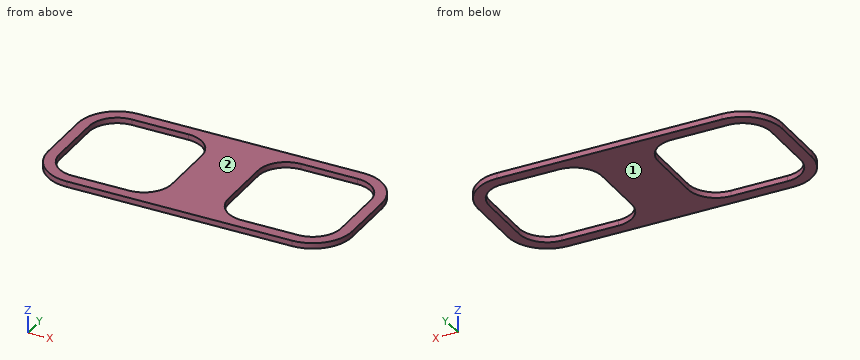
```python
from build123d import *

# Parameters (mm, degrees)
F1_DEPTH = 0.5


with BuildPart() as f1:
    # F0 (on Top) → F1 (new body)
    with BuildSketch(Plane.XY):
        with BuildLine():
            Line((-13.5, 2.5), (-13.5, 0))
            Line((-13.5, 0), (-13.5, -2.5))
            ThreePointArc((-13.5, -2.5), (-12.474874, -4.974874), (-10, -6))
            Line((-10, -6), (10, -6))
            ThreePointArc((10, -6), (12.474874, -4.974874), (13.5, -2.5))
            Line((13.5, -2.5), (13.5, 2.5))
            ThreePointArc((13.5, 2.5), (12.474874, 4.974874), (10, 6))
            Line((10, 6), (-10, 6))
            ThreePointArc((-10, 6), (-12.474874, 4.974874), (-13.5, 2.5))
        make_face()
        with BuildLine():
            Line((-2.5, 2.5), (-2.5, 0))
            Line((-2.5, 0), (-2.5, -2.5))
            ThreePointArc((-2.5, -2.5), (-3.232233, -4.267767), (-5, -5))
            Line((-5, -5), (-10, -5))
            ThreePointArc((-10, -5), (-11.767767, -4.267767), (-12.5, -2.5))
            Line((-12.5, -2.5), (-12.5, 0))
            Line((-12.5, 0), (-12.5, 2.5))
            ThreePointArc((-12.5, 2.5), (-11.767767, 4.267767), (-10, 5))
            Line((-10, 5), (-5, 5))
            ThreePointArc((-5, 5), (-3.232233, 4.267767), (-2.5, 2.5))
        make_face(mode=Mode.SUBTRACT)
        with BuildLine():
            Line((2.5, -2.5), (2.5, 0))
            Line((2.5, 0), (2.5, 2.5))
            ThreePointArc((2.5, 2.5), (3.232233, 4.267767), (5, 5))
            Line((5, 5), (10, 5))
            ThreePointArc((10, 5), (11.767767, 4.267767), (12.5, 2.5))
            Line((12.5, 2.5), (12.5, -2.5))
            ThreePointArc((12.5, -2.5), (11.767767, -4.267767), (10, -5))
            Line((10, -5), (5, -5))
            ThreePointArc((5, -5), (3.232233, -4.267767), (2.5, -2.5))
        make_face(mode=Mode.SUBTRACT)
    extrude(amount=F1_DEPTH)


solid = f1.part
```
Read the model definition and answer for the solid it produces. Units are mm, in the model's axes. Face numbers are marked on the shaded views. Round coordinates to 2 decimals unless told otherwise and drop trailing zeros. Write each loop counter-clockwise with the first axis right and the second up, starting at its lowest first coordinate (ties: lowest second). Pieces come first, ordered by that corner, then holes. Notation, with made-up numbers: (0.25, -5.5) -> (42.25, -5.5) arc R25 ccw to (42.25, 24.5) -> close; hole circle Ø10 at (79.5, 37). An arc over 180 degrees is marked (long way). Answer in a Markdown table with one row per item. Add a question column.
1) Find section B-B, the plane y = 0.5. Determine the outline of the cut face in (x, z).
2) Determine the mould class of the marked faces 1 and 2 for opening direction Z: pulls with the +Z half, pulls with the -Z half, needs draft (parallel to the pull), parting line crosses it, or undercut.
3) Find section C-C, the plane z = 0.4. Determine the outline of the cut face in (x, y).
4) Find section D-D, the plane y = 3.5. Determine the outline of the cut face in (x, z).
5) Consider line 1 (X direction, y = -1.25, z = 0.3); line 2 (Y direction, x = 7.75, z = 0.1); line 3 (X direction, y = -3.5, z = 0.1). Determine where each line is inside the solid, lowest interval first.
6) Find section A-A, the plane x = -7.5. Determine the outline of the cut face in (y, z), and give its area (3 significant figures).
Findings below:
| question | item | result |
|---|---|---|
| 1 | outline | (-13.5, 0) -> (-12.5, 0) -> (-12.5, 0.5) -> (-13.5, 0.5) -> close; (-2.5, 0) -> (2.5, 0) -> (2.5, 0.5) -> (-2.5, 0.5) -> close; (12.5, 0) -> (13.5, 0) -> (13.5, 0.5) -> (12.5, 0.5) -> close |
| 2 | face 1 | pulls with the -Z half |
| 2 | face 2 | pulls with the +Z half |
| 3 | outline | (-13.5, -2.5) arc R3.5 ccw to (-10, -6) -> (10, -6) arc R3.5 ccw to (13.5, -2.5) -> (13.5, 2.5) arc R3.5 ccw to (10, 6) -> (-10, 6) arc R3.5 ccw to (-13.5, 2.5) -> close; hole (-12.5, -2.5) arc R2.5 ccw to (-10, -5) -> (-5, -5) arc R2.5 ccw to (-2.5, -2.5) -> (-2.5, 2.5) arc R2.5 ccw to (-5, 5) -> (-10, 5) arc R2.5 ccw to (-12.5, 2.5) -> close; hole (2.5, -2.5) arc R2.5 ccw to (5, -5) -> (10, -5) arc R2.5 ccw to (12.5, -2.5) -> (12.5, 2.5) arc R2.5 ccw to (10, 5) -> (5, 5) arc R2.5 ccw to (2.5, 2.5) -> close |
| 4 | outline | (-13.35, 0) -> (-12.29, 0) -> (-12.29, 0.5) -> (-13.35, 0.5) -> close; (-2.71, 0) -> (2.71, 0) -> (2.71, 0.5) -> (-2.71, 0.5) -> close; (12.29, 0) -> (13.35, 0) -> (13.35, 0.5) -> (12.29, 0.5) -> close |
| 5 | line 1 | -13.5 to -12.5, -2.5 to 2.5, 12.5 to 13.5 |
| 5 | line 2 | -6 to -5, 5 to 6 |
| 5 | line 3 | -13.35 to -12.29, -2.71 to 2.71, 12.29 to 13.35 |
| 6 | outline | (-6, 0) -> (-5, 0) -> (-5, 0.5) -> (-6, 0.5) -> close; (5, 0) -> (6, 0) -> (6, 0.5) -> (5, 0.5) -> close |
| 6 | area | 1.00 mm² |
